from build123d import *

# Parameters (mm, degrees)
SKETCH1_W           = 105.6
SKETCH1_H           = 57.3
BOSS_EXTRUDE1_DEPTH = 3
SKETCH1_4_R         = 2.45
SKETCH1_4_R_2       = 1.45
BOSS_EXTRUDE2_DEPTH = 6


with BuildPart() as part:
    # Sketch1 → Boss-Extrude1 (new body)
    with BuildSketch(Plane(origin=(0, 0, 0), x_dir=(1, 0, 0), z_dir=(0, 1, 0))):
        with Locations((50.8, 26.65)):
            Rectangle(SKETCH1_W, SKETCH1_H)
    extrude(amount=-BOSS_EXTRUDE1_DEPTH)

    # Sketch1_4 → Boss-Extrude2 (add)
    with BuildSketch(Plane(origin=(0, 0, 0), x_dir=(1, 0, 0), z_dir=(0, 1, 0))):
        with Locations(Location((13.97, 2.54, 0), (0, 0, 270))):  # turned: the seam where the file's is
            Circle(SKETCH1_4_R)
        with Locations(Location((13.97, 2.54, 0), (0, 0, 270))):  # turned: the seam where the file's is
            Circle(SKETCH1_4_R_2, mode=Mode.SUBTRACT)
        with Locations(Location((15.24, 50.8, 0), (0, 0, 270))):  # turned: the seam where the file's is
            Circle(SKETCH1_4_R)
        with Locations(Location((15.24, 50.8, 0), (0, 0, 270))):  # turned: the seam where the file's is
            Circle(SKETCH1_4_R_2, mode=Mode.SUBTRACT)
        with Locations(Location((66.04, 35.56, 0), (0, 0, 270))):  # turned: the seam where the file's is
            Circle(SKETCH1_4_R)
        with Locations(Location((66.04, 35.56, 0), (0, 0, 270))):  # turned: the seam where the file's is
            Circle(SKETCH1_4_R_2, mode=Mode.SUBTRACT)
        with Locations(Location((66.04, 7.62, 0), (0, 0, 270))):  # turned: the seam where the file's is
            Circle(SKETCH1_4_R)
        with Locations(Location((66.04, 7.62, 0), (0, 0, 270))):  # turned: the seam where the file's is
            Circle(SKETCH1_4_R_2, mode=Mode.SUBTRACT)
        with Locations(Location((96.52, 2.54, 0), (0, 0, 270))):  # turned: the seam where the file's is
            Circle(SKETCH1_4_R)
        with Locations(Location((96.52, 2.54, 0), (0, 0, 270))):  # turned: the seam where the file's is
            Circle(SKETCH1_4_R_2, mode=Mode.SUBTRACT)
        with Locations(Location((90.17, 50.8, 0), (0, 0, 270))):  # turned: the seam where the file's is
            Circle(SKETCH1_4_R)
        with Locations(Location((90.17, 50.8, 0), (0, 0, 270))):  # turned: the seam where the file's is
            Circle(SKETCH1_4_R_2, mode=Mode.SUBTRACT)
    extrude(amount=BOSS_EXTRUDE2_DEPTH)


solid = part.part
Build history of the part. All positions in model axes, mm. A direction names the side the tool comes from. Coordinates: 2 decimals unless noted, no trailing zeros. Write each loop counter-clockwise with the first axis right and the second up, starting at its lowest first coordinate (ties: lowest second). Pieces come first, ordered by that corner, then holes. Notation, with made-up numbers: (-5.5, -36) -> (26.5, -36) arc R19 ccw to (26.5, -11) -> close; hole circle Ø4 at (-10, -38). An arc over 180 degrees is marked (long way). Use CSV: the item, a comma, the result in double quotes. Start each with the question number.
Q1. Cut at D-D, the plane z = -50.8. List the corners of the cut face in (x, y).
Q2. Cut at B-B, the plane z = -35.56. List the corners of the cut face in (x, y), then the cut area to 3 significant figures.
Q3. Pull direction X, two halves, no side cores. Call faces 3 (the flat face through (103.6, -1, -26)), 4 (the flat face through (95, 6, -1)), 5 (the cylindrical face through (15.348, 2.958, -53.248)), 6 (the cylindrical face through (68.47, 2.96, -7.94)): released by +X, released by -X, zero draft, split by the parting line, or undercut.
Q4. Drill centre lines: probe 1 along X at (y, z) = (4.3, -2.54); probe 2 along X at (y, z) = (2.3, -50.8); probe 3 along X at (y, z) = (4.55, -7.62). Where is each one in solid material? Low to high.
Q5. Cut at A-A, the plane y = 2. State how many separate pieces and enclosed holes the cut face has, then the cut area to 3 significant figures.
Q6. Cut at C-C, the plane x = 90.17. List the corners of the cut face in (y, z).
Q7. 3-axis set-ups, long thin cutter, end or side, ignore diameter. For faces 1 (the flat face through (66, 0, -36)), 2 (the flat face through (50, -1, 2)): which of +Z, -Z, +X, -X, +Y, -Y reach the whole face in a straight line?
Q8. Flat gauge pins, fed straight in: pin 1 Ø1.7 at (x, z) = (66.04, -7.62) entering from +Y; pin 2 Ø1 at (x, y) = (66.5, 4) entering from +Z. Where does each tip first touch, or does it go through?
Checked values:
1,outline,"(-2, -3) -> (103.6, -3) -> (103.6, 0) -> (92.62, 0) -> (92.62, 6) -> (91.62, 6) -> (91.62, 0) -> (88.72, 0) -> (88.72, 6) -> (87.72, 6) -> (87.72, 0) -> (17.69, 0) -> (17.69, 6) -> (16.69, 6) -> (16.69, 0) -> (13.79, 0) -> (13.79, 6) -> (12.79, 6) -> (12.79, 0) -> (-2, 0) -> close"
2,outline,"(-2, -3) -> (103.6, -3) -> (103.6, 0) -> (68.49, 0) -> (68.49, 6) -> (67.49, 6) -> (67.49, 0) -> (64.59, 0) -> (64.59, 6) -> (63.59, 6) -> (63.59, 0) -> (-2, 0) -> close"
2,area,"329 mm²"
3,face 3,"released by +X"
3,face 4,"zero draft"
3,face 5,"undercut"
3,face 6,"split by the parting line"
4,probe 1,"x = 11.52 to 12.52, 15.42 to 16.42, 94.07 to 95.07, 97.97 to 98.97"
4,probe 2,"x = 12.79 to 13.79, 16.69 to 17.69, 87.72 to 88.72, 91.62 to 92.62"
4,probe 3,"x = 63.59 to 64.59, 67.49 to 68.49"
5,separate pieces,"6"
5,enclosed holes,"6"
5,area,"73.5 mm²"
6,outline,"(-3, -55.3) -> (0, -55.3) -> (0, -53.25) -> (6, -53.25) -> (6, -52.25) -> (0, -52.25) -> (0, -49.35) -> (6, -49.35) -> (6, -48.35) -> (0, -48.35) -> (0, 2) -> (-3, 2) -> close"
7,face 1,"+Y"
7,face 2,"+Z, +X, -X, +Y, -Y"
8,pin 1,"stops at y = 0"
8,pin 2,"stops at z = -5.17"
